Input: part model. Units: mm. Frame: model coordinates. Face numbers are marked on the shaded views. A direction names the side the tool comes from. Coordinates: 2 decimals unless noted, no trailing zeros. Write each loop counter-clockwise with the first axis right and the second up, starting at its lowest first coordinate (ties: lowest second). Pieces come first, ordered by that corner, then holes. Notation, with made-up numbers: (78, 75.25) -> (91, 75.25) arc R21 cw to (91, 94.25) -> close; hole circle Ø10 at (-36, -0.75). An arc over 180 degrees is marked (long way). Use one line per item in the form item = value. Start each with the question number.
(1) Cut plane D-D on z = 15.5. Return the cut outline in (x, y).
(2) Set-up query: the marked faces 1 and 2. Return all of +Z, -Z, +X, -X, +Y, -Y with unobstructed straight access to the full face (end or side cutting, diameter ignored); none if empty.
(3) Pull-direction query (Z, two-part tool) for the marked faces 3, 4, 5 and 6; classes: released by +Z, released by -Z, zero draft, split by the parting line, or undercut.
(4) Cut plane A-A on x = -5.75. State how many separate pieces and enclosed holes the cut face has, plus the area to 3 significant figures.
(5) First-contact query: pin 1 (10 mm diameter, centred on y = -6.5, z = 19, fed in from -X); pin 2 (3 mm diameter, centred on x = -5.5, y = 7, fed in from +Z); pin 3 (1 mm diameter, centred on x = -1.5, z = -1, fed in from -Y). Flat tips, straight axial feed; report the tip coordinate or a pass-through.
(6) Ray query, line 1 along Z through (x, y) = (-0.55, 0) (1 decimal); line 2 along Z through (x, y) = (-2, 0) (1 decimal); line 3 along Z through (x, y) = (-3.5, -7.75). Return the intervals inside material, ascending.
(7) Cut plane B-B on z = 9. Return the cut outline in (x, y), plus the area to 3 significant figures.
```python
from build123d import *

# Parameters (mm, degrees)
F0_W      = 4.7625
F0_H      = 12.7
F1_ANGLE  = 180
F2_R      = 1.5875
F3_DEPTH  = 3.175
F4_R      = 0.508
F1_FACE_R = 1.5875
F5_DEPTH  = 0.127


with BuildPart() as f1:
    # F0 (on Right) → F1 (revolve)
    with BuildSketch(Plane.YZ):
        with BuildLine():
            Line((0, 31.75), (0, 0))
            Line((0, 0), (4.7625, 0))
            Line((4.7625, 0), (9.525, 0))
            Line((9.525, 0), (9.525, 3.175))
            Line((9.525, 3.175), (7.9375, 4.7625))
            ThreePointArc((7.9375, 4.7625), (9.171707, 5.725409), (9.504834, 7.254947))
            ThreePointArc((9.504834, 7.254947), (4.867571, 10.849768), (3.175, 16.467789))
            Line((3.175, 16.467789), (6.35, 16.467789))
            Line((6.35, 16.467789), (6.35, 18.317595))
            Line((6.35, 18.317595), (2.46587, 22.459295))
            ThreePointArc((2.46587, 22.459295), (4.806186, 28.053033), (0, 31.75))
        make_face()
        with Locations((2.38125, -6.35)):
            Rectangle(F0_W, F0_H)
        Polygon((4.7625, -12.7), (0, -12.7), (0, -15.875), (6.35, -15.875), align=None)
    revolve(axis=Axis((0, 0, 15.875), (0, 0, 1)), revolution_arc=F1_ANGLE)

    # F2 (on face) → F3 (cut)
    with BuildSketch(Plane.YZ):
        with Locations((0, 3.175)):
            Circle(F2_R)
        with Locations((0, -9.525)):
            Circle(F2_R)
    extrude(amount=-F3_DEPTH, mode=Mode.SUBTRACT)

    # F4
    f4_edges = [f1.edges().sort_by_distance(p)[0] for p in [
        (-3.175, 0, 16.467789),
    ]]
    fillet(f4_edges, radius=F4_R)

    # F1_face (on face) → F5 (join)
    with BuildSketch(Plane(origin=(0, 0, 6.530127), x_dir=(0, 1, 0), z_dir=(1, 0, 0))):
        with BuildLine():
            Line((3.688236, 9.937662), (6.35, 9.937662))
            Line((6.35, 9.937662), (6.35, 11.787469))
            Line((6.35, 11.787469), (2.46587, 15.929168))
            ThreePointArc((2.46587, 15.929168), (4.806186, 21.522907), (0, 25.219873))
            ThreePointArc((0, 25.219873), (-4.806186, 21.522907), (-2.46587, 15.929168))
            Line((-2.46587, 15.929168), (-6.35, 11.787469))
            Line((-6.35, 11.787469), (-6.35, 9.937662))
            Line((-6.35, 9.937662), (-3.688236, 9.937662))
            add(Edge.make_bspline(
                [(-3.688236, 9.937662), (-3.657727, 9.937662), (-3.626288, 9.935464), (-3.594162, 9.930815), (-3.561678, 9.923496), (-3.529253, 9.913372), (-3.465394, 9.887476), (-3.433961, 9.871702), (-3.40348, 9.85309), (-3.374427, 9.831747), (-3.347244, 9.807928), (-3.297392, 9.756145), (-3.274705, 9.728198), (-3.254541, 9.698489), (-3.237138, 9.667463), (-3.222581, 9.635595), (-3.199016, 9.570815), (-3.190049, 9.537897), (-3.183914, 9.505022), (-3.180455, 9.472607), (-3.17944, 9.440977), (-3.180603, 9.410368)],
                knots=[0, 0, 0, 0, 0, 0, 0, 0.24993, 0.24993, 0.24993, 0.24993, 0.24993, 0.5, 0.5, 0.5, 0.5, 0.5, 0.74907, 0.74907, 0.74907, 0.74907, 0.74907, 1, 1, 1, 1, 1, 1, 1], degree=6))
            ThreePointArc((-3.180603, 9.410368), (-5.019853, 4.104372), (-9.504834, 0.72482))
            ThreePointArc((-9.504834, 0.72482), (-9.171707, -0.804718), (-7.9375, -1.767627))
            Line((-7.9375, -1.767627), (-9.525, -3.355127))
            Line((-9.525, -3.355127), (-9.525, -6.530127))
            Line((-9.525, -6.530127), (-4.7625, -6.530127))
            Line((-4.7625, -6.530127), (-4.7625, -19.230127))
            Line((-4.7625, -19.230127), (-6.35, -22.405127))
            Line((-6.35, -22.405127), (6.35, -22.405127))
            Line((6.35, -22.405127), (4.7625, -19.230127))
            Line((4.7625, -19.230127), (4.7625, -6.530127))
            Line((4.7625, -6.530127), (9.525, -6.530127))
            Line((9.525, -6.530127), (9.525, -3.355127))
            Line((9.525, -3.355127), (7.9375, -1.767627))
            ThreePointArc((7.9375, -1.767627), (9.171707, -0.804718), (9.504834, 0.72482))
            ThreePointArc((9.504834, 0.72482), (5.019853, 4.104372), (3.180603, 9.410368))
            add(Edge.make_bspline(
                [(3.688236, 9.937662), (3.657727, 9.937662), (3.626288, 9.935464), (3.594162, 9.930815), (3.561678, 9.923496), (3.529253, 9.913372), (3.465394, 9.887476), (3.433961, 9.871702), (3.40348, 9.85309), (3.374427, 9.831747), (3.347244, 9.807928), (3.297392, 9.756145), (3.274705, 9.728198), (3.254541, 9.698489), (3.237138, 9.667463), (3.222581, 9.635595), (3.199016, 9.570815), (3.190049, 9.537897), (3.183914, 9.505022), (3.180455, 9.472607), (3.17944, 9.440977), (3.180603, 9.410368)],
                knots=[0, 0, 0, 0, 0, 0, 0, 0.24993, 0.24993, 0.24993, 0.24993, 0.24993, 0.5, 0.5, 0.5, 0.5, 0.5, 0.74907, 0.74907, 0.74907, 0.74907, 0.74907, 1, 1, 1, 1, 1, 1, 1], degree=6))
        make_face()
        with Locations((0, -16.055127)):
            Circle(F1_FACE_R, mode=Mode.SUBTRACT)
        with Locations((0, -3.355127)):
            Circle(F1_FACE_R, mode=Mode.SUBTRACT)
    extrude(amount=F5_DEPTH)


solid = f1.part
```
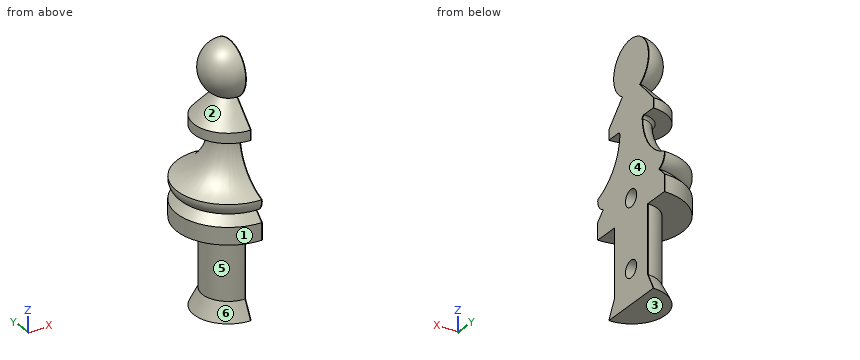
Values:
q1.outline = (0, -3.21) -> (0.13, -3.21) -> (0.13, 3.21) -> (0, 3.21) arc R3.21 ccw to start
q2.face_1 = +Z, -Z, -X
q2.face_2 = -X
q3.face_3 = released by -Z
q3.face_4 = zero draft
q3.face_5 = undercut
q3.face_6 = undercut
q4.separate_pieces = 3
q4.enclosed_holes = 0
q4.area = 142 mm2
q5.pin_1 = -6.16
q5.pin_2 = 8.33
q5.pin_3 = -4.66
q6.line_1 = -15.9 to -11.1, -7.9 to 1.6, 4.8 to 31.7
q6.line_2 = -15.9 to -11.1, -7.9 to 1.6, 4.8 to 31.3
q6.line_3 = 0 to 4.2, 5.04 to 7.69
q7.outline = (0, -6.53) -> (0.13, -6.53) -> (0.13, 6.53) -> (0, 6.53) arc R6.53 ccw to start
q7.area = 68.6 mm2
